Geometry: final body of the model. Coordinates: model frame, mm. A direction names the side the tool comes from. Coordinates: 2 decimals unless noted, no trailing zeros. Order: outer loops, then holes, each group sorted by start corner. A loop starts at its lowest first (then second) coordinate and runs counter-clockwise, first axis right, second up. Notation, with made-up numbers: (40, -33.5) - (95, -33.5) arc R5 cw to (95, -26.5) - close; hole circle Ø11 at (88, -21). An arc over 180 degrees is marked (long way). Use a Markdown table: item, result. Add a question column.
```python
from build123d import *

# Parameters (mm, degrees)
EXTRUDE1_DEPTH = 60
EXTRUDE2_DEPTH = 95.991377429
EXTRUDE3_DEPTH = 100
EXTRUDE4_DEPTH = 100


with BuildPart() as part:
    # Sketch1 → Extrude1 (new body)
    with BuildSketch(Plane(origin=(0, 0, 0), x_dir=(1, 0, 0), z_dir=(0, 1, 0))):
        Polygon((0, 0), (-50.143211133, 48.843201956), (-15.255209736, 84.659781336), (34.888001397, 35.816579381), align=None)
    extrude(amount=EXTRUDE1_DEPTH)

    # Sketch2 → Extrude2 (cut, through all)
    with BuildSketch(Plane(origin=(0, 0, 0), x_dir=(0.697760028, 0, -0.716331588), z_dir=(0.716331588, 0, 0.697760028))):
        Polygon((50, 60), (0, 30), (0, 60), align=None)
    extrude(amount=-EXTRUDE2_DEPTH, mode=Mode.SUBTRACT)

    # Sketch3 → Extrude3 (add)
    with BuildSketch(Plane(origin=(0, 0, 0), x_dir=(1, 0, 0), z_dir=(0, 1, 0))):
        Polygon((20.932800838, 21.489947628), (3.024511148, 38.933948327), (58.845313383, 96.240475336), (94.661892763, 61.352473939), (52.796291087, 18.372578682), (34.888001397, 35.816579381), align=None)
    extrude(amount=EXTRUDE3_DEPTH)

    # Sketch4 → Extrude4 (cut)
    with BuildSketch(Plane(origin=(20.932800838, 0, -21.489947628), x_dir=(0.716331588, 0, 0.697760028), z_dir=(-0.697760028, 0, 0.716331588))):
        Polygon((25, 60), (-25, 100), (25, 100), align=None)
    extrude(amount=-EXTRUDE4_DEPTH, mode=Mode.SUBTRACT)


solid = part.part
```
1) Set-up query: faces 4 (the face through (48.703, 79.72, -49.498)), 5 (the face through (43.97, 30.55, -26.97)), 6 (the face through (12.104, 67.858, -30.09)). Return all of +Z, -Z, +X, -X, +Y, -Y with unobstructed straight access to the full face (end or side cutting, diameter ignored); none if empty.
2) Section A-A (z = -79). Return loops of the section in (x, y), then the cut area to 3 significant figures.
3) Section C-C (x = 7). Return loops of the section in (y, z).
4) Ray query, line 1 along X through (y, z) = (41.5, -68); line 2 along X through (y, z) = (5, -65); line 3 along Y through (x, z) = (63, -42). Return the intervals inside material, ascending.
5) Section B-B (y = 11). Return loops of the section in (x, z).
6) Pin query (flat end, axial travel): pin 1 (1.5 mm diameter, centred on y = 20, z = -13, fed in from +X); pin 2 (5 mm diameter, centred on x = -1, y = 16, fed in from -Z); pin 3 (4 mm diameter, centred on x = 26.5, y = 39.5, fed in from +Z). Return the tip coordinate at first contact, or that it passes through.
7) Section D-D (z = -66.5). Return loops of the section in (x, y).
8) Draft query along X for faces 1 (the face through (74.02, 29.58, -40.16)), 2 (the face through (-32.943, 22.913, -66.501)), 3 (the face through (0.637, 29.58, -69.18)). Return one class per face: pulls with the +X half, pulls with the -X half, needs draft (parallel to the pull), parting line crosses it, or undercut.
Values follow:
| question | item | result |
|---|---|---|
| 1 | face 4 | +Z, +X, +Y |
| 1 | face 5 | +Z, +Y, -Y |
| 1 | face 6 | +Z, -X, +Y |
| 2 | outline | (-20.77, 0) - (-9.44, 0) - (-9.44, 60) - (-20.77, 55.26) - close; (42.05, 0) - (76.54, 0) - (76.54, 80.23) - (42.05, 100) - close |
| 2 | area | 3,760 mm² |
| 3 | outline | (0, -62.98) - (60, -62.98) - (51.42, -43.02) - (100, -43.02) - (95.56, -35.06) - (48, -35.06) - (36.02, -7.19) - (0, -7.19) - close |
| 4 | line 1 | x = -31.48 to 1.85, 31.34 to 87.84 |
| 4 | line 2 | x = -34.41 to 4.93, 28.41 to 90.92 |
| 4 | line 3 | y = 0 to 67.34 |
| 5 | outline | (-50.14, -48.84) - (-15.26, -84.66) - (16.98, -53.26) - (58.85, -96.24) - (94.66, -61.35) - (52.8, -18.37) - (34.89, -35.82) - (0, 0) - close |
| 6 | pin 1 | stops at x = 13.39 |
| 6 | pin 2 | stops at z = -73.21 |
| 6 | pin 3 | stops at z = -25.15 |
| 7 | outline | (-32.94, 0) - (3.39, 0) - (3.39, 60) - (-32.94, 44.79) - close; (29.88, 0) - (89.38, 0) - (89.38, 65.9) - (29.88, 100) - close |
| 8 | face 1 | pulls with the +X half |
| 8 | face 2 | pulls with the -X half |
| 8 | face 3 | undercut |
